from build123d import *

# Parameters (mm, degrees)
SKETCH1_W            = 175
SKETCH1_H            = 24
BOSS_EXTRUDE3_DEPTH  = 10
SKETCH1_6_R          = 20
SKETCH1_6_R_2        = 10
HEAD_WIDTH_DEPTH     = 19
SKETCH1_7_R          = 20
SKETCH1_7_R_2        = 10
CUT_EXTRUDE1_DEPTH   = 6.25
FILLET1_START        = -6.25
FILLET1_DEPTH        = 12.5
FILLET2_R            = 3.25
SKETCH2_W            = 158.5
SKETCH2_H            = 14
CUT_EXTRUDE2_DEPTH   = 5
FILLET3_R            = 5
FILLET3_OF_MIRROR1_R = 5


with BuildPart() as part:
    # Sketch1 → Boss-Extrude3 (new, symmetric)
    with BuildSketch(Plane.XY):
        with Locations((125, 0)):
            Rectangle(SKETCH1_W, SKETCH1_H)
    extrude(amount=BOSS_EXTRUDE3_DEPTH, both=True)

    # Sketch1<6> → Head Width (add, symmetric)
    # profile 1 of 4: a face of its own
    with BuildSketch(Plane.XY):
        with BuildLine():
            Line((37.5, -12), (37.5, 12))
            Line((37.5, 12), (37.5, 20))
            Line((37.5, 20), (0, 20))
            ThreePointArc((0, 20), (14.142135624, 14.142135624), (20, 0))
            ThreePointArc((20, 0), (14.142135624, -14.142135624), (0, -20))
            Line((0, -20), (37.5, -20))
            Line((37.5, -20), (37.5, -12))
        make_face()
    # profile 2 of 4: a face of its own
    with BuildSketch(Plane.XY):
        Circle(SKETCH1_6_R)
        Circle(SKETCH1_6_R_2, mode=Mode.SUBTRACT)
    # profile 3 of 4: a face of its own
    with BuildSketch(Plane.XY):
        with BuildLine():
            Line((212.5, 20), (212.5, 12))
            Line((212.5, 12), (212.5, -12))
            Line((212.5, -12), (212.5, -20))
            Line((212.5, -20), (250, -20))
            ThreePointArc((250, -20), (230, 0), (250, 20))
            Line((250, 20), (212.5, 20))
        make_face()
    # profile 4 of 4: a face of its own
    with BuildSketch(Plane.XY):
        with Locations((250, 0)):
            Circle(SKETCH1_6_R)
        with Locations((250, 0)):
            Circle(SKETCH1_6_R_2, mode=Mode.SUBTRACT)
    extrude(amount=HEAD_WIDTH_DEPTH, both=True)

    # Sketch1<7> → Cut-Extrude1 (cut, symmetric)
    # profile 1 of 2: a face of its own
    with BuildSketch(Plane.XY):
        Circle(SKETCH1_7_R)
        Circle(SKETCH1_7_R_2, mode=Mode.SUBTRACT)
    # profile 2 of 2: a face of its own
    with BuildSketch(Plane.XY):
        with Locations((250, 0)):
            Circle(SKETCH1_7_R)
        with Locations((250, 0)):
            Circle(SKETCH1_7_R_2, mode=Mode.SUBTRACT)
    extrude(amount=CUT_EXTRUDE1_DEPTH, both=True, mode=Mode.SUBTRACT)

    # Fillet1: read off the stored shape, not the designer's step
    # Fillet1 outline → Fillet1 (cut)
    with BuildSketch(Plane.XY.offset(FILLET1_START)):
        with BuildLine():
            ThreePointArc((230, 20), (234.472135955, 17.236067977), (234, 12))
            ThreePointArc((234, 12), (241.05572809, 17.88854382), (250, 20))
            Line((250, 20), (230, 20))
        make_face()
        with BuildLine():
            ThreePointArc((234, -12), (234.472135955, -17.236067977), (230, -20))
            Line((230, -20), (250, -20))
            ThreePointArc((250, -20), (241.05572809, -17.88854382), (234, -12))
        make_face()
        with BuildLine():
            ThreePointArc((20, -20), (15.527864045, -17.236067977), (16, -12))
            ThreePointArc((16, -12), (8.94427191, -17.88854382), (0, -20))
            Line((0, -20), (20, -20))
        make_face()
        with BuildLine():
            ThreePointArc((0, 20), (8.94427191, 17.88854382), (16, 12))
            ThreePointArc((16, 12), (15.527864045, 17.236067977), (20, 20))
            Line((20, 20), (0, 20))
        make_face()
    extrude(amount=FILLET1_DEPTH, mode=Mode.SUBTRACT)

    # Fillet2
    fillet2_edges = [part.edges().sort_by_distance(p)[0] for p in [
        (37.5, 0, 10),
        (37.5, 20, 0),
        (37.5, 0, 19),
        (37.5, -20, 0),
        (37.5, 0, -19),
        (212.5, -20, 0),
        (212.5, 0, -19),
        (212.5, 20, 0),
        (212.5, 0, 19),
        (212.5, 0, 10),
        (37.5, 0, -10),
        (212.5, 0, -10),
        (212.5, -12, 0),
        (37.5, -12, 0),
        (37.5, 12, 0),
        (212.5, 12, 0),
    ]]
    fillet(fillet2_edges, radius=FILLET2_R)

    # Sketch2 → Cut-Extrude2 (cut)
    with BuildSketch(Plane.XY.offset(10)):
        with Locations((125, 0)):
            Rectangle(SKETCH2_W, SKETCH2_H)
    cut_extrude2 = extrude(amount=-CUT_EXTRUDE2_DEPTH, mode=Mode.SUBTRACT)

    # Fillet3
    fillet3_edges = [part.edges().sort_by_distance(p)[0] for p in [
        (45.75, -7, 7.5),
        (45.75, 7, 7.5),
        (204.25, 7, 7.5),
        (204.25, -7, 7.5),
    ]]
    fillet(fillet3_edges, radius=FILLET3_R)

    # Mirror1: Cut-Extrude2 across plane
    add(cut_extrude2.mirror(Plane.XY), mode=Mode.SUBTRACT)

    # Fillet3 of Mirror1
    fillet3_of_mirror1_edges = [part.edges().sort_by_distance(p)[0] for p in [
        (45.75, -7, -7.5),
        (45.75, 7, -7.5),
        (204.25, 7, -7.5),
        (204.25, -7, -7.5),
    ]]
    fillet(fillet3_of_mirror1_edges, radius=FILLET3_OF_MIRROR1_R)


solid = part.part
Source: CAD feature listing. Evaluate the final solid. Frame: model axes, mm. A direction names the side the tool comes from. Round coordinates to 2 decimals unless told otherwise and drop trailing zeros. Order: outer loops, then holes, each group sorted by start corner. A loop starts at its lowest first (then second) coordinate and runs counter-clockwise, first axis right, second up. Notation, with made-up numbers: (-38.75, 87) - (-6.75, 87) arc R19 cw to (-6.75, 115) - close; hole circle Ø7 at (-7, 70). An arc over 180 degrees is marked (long way). Use a Markdown table: item, result. Add a question column.
1. First-contact query: pin 1 (23 mm diameter, centred on x = 250, y = 0, fed in from +Z); pin 2 (2 mm diameter, centred on x = 178, y = -5.5, fed in from -Z); pin 3 (12 mm diameter, centred on y = -15, z = 10, fed in from +X); pin 4 (4.5 mm diameter, centred on y = -0.5, z = -8, fed in from +X). Flat tips, straight axial feed; report the tip coordinate or a pass-through.
2. Section query A-A (x = 159.5). Return the cut outline in (y, z).
3. Set-up query: faces 5 (the cylindrical face through (202.82, 5.5, -7.46)), 6 (the cylindrical face through (15.494, 17.166, -0.088)), 7 (the flat face through (124, 12, 0)), 8 (the cylindrical face through (230, 0, 0)), 9 (the flat face through (37.5, -1, 14)). Return all of +Z, -Z, +X, -X, +Y, -Y with unobstructed straight access to the full face (end or side cutting, diameter ignored); none if empty.
4. Mould query, pull axis Y, two halves, no side actions, for faces 1 (the cylindrical face through (20, 0, 0)), 2 (the flat face through (124, -12, 0)), 3 (the flat face through (124, 0, 5)), 4 (the cylindrical face through (-20, 0, 13)). Classes: +Y half, -Y half, draft (parallel to the pull), parting line (faces both ways), or undercut.
5. Line query: probe 1 along Y at (x, z) = (0, -15.75); probe 2 along Y at (x, z) = (47.5, 9.5); probe 3 along Z at (x, y) = (203.5, 9). Output: solid intervals per line, ascending.
Derived:
| question | item | result |
|---|---|---|
| 1 | pin 1 | z = 19 |
| 1 | pin 2 | z = -5 |
| 1 | pin 3 | x = 267.86 |
| 1 | pin 4 | x = 270 |
| 2 | outline | (-12, -10) - (-7, -10) - (-7, -5) - (7, -5) - (7, -10) - (12, -10) - (12, 10) - (7, 10) - (7, 5) - (-7, 5) - (-7, 10) - (-12, 10) - close |
| 3 | face 5 | -Z |
| 3 | face 6 | -X |
| 3 | face 7 | +Z, -Z, +Y |
| 3 | face 8 | +X |
| 3 | face 9 | none |
| 4 | face 1 | undercut |
| 4 | face 2 | -Y half |
| 4 | face 3 | undercut |
| 4 | face 4 | parting line |
| 5 | probe 1 | -20 to -10, 10 to 20 |
| 5 | probe 2 | -12 to -5.8, 5.8 to 12 |
| 5 | probe 3 | -10 to 10 |
